```python
from build123d import *

# Parameters (mm, degrees)
BOSS_EXTRUDE1_DEPTH = 4.064


with BuildPart() as part:
    # Sketch1 → Boss-Extrude1 (new body)
    with BuildSketch(Plane(origin=(0, 0, 0), x_dir=(0, 0, -1), z_dir=(1, 0, 0))):
        Polygon((10.353307799, 10.287), (10.353307799, 0), (33.467307799, 0), (33.467307799, 2.413), (30.292307799, 2.413), (30.292307799, 3.937), (33.467307799, 3.937), (33.467307799, 7.493), (30.292307799, 7.493), (30.292307799, 10.287), align=None)
        Polygon((-12.760692201, 2.413), (-12.760692201, 0), (10.353307799, 0), (10.353307799, 10.287), (-9.585692201, 10.287), (-9.585692201, 7.493), (-12.760692201, 7.493), (-12.760692201, 3.937), (-9.585692201, 3.937), (-9.585692201, 2.413), align=None)
    extrude(amount=BOSS_EXTRUDE1_DEPTH)


solid = part.part
```
The listing builds one solid part. Answer for the finished solid, in the listing's coordinates (mm). A direction names the side the tool comes from. Coordinates: 2 decimals unless noted, no trailing zeros. Loops run counter-clockwise (first coordinate to the right, second up) from the corner with the lowest first, then second, coordinate; pieces in that order, holes last. Notation, with made-up numbers: (53, 55.25) - (65, 55.25) arc R18 ccw to (65, 78.25) - close; hole circle Ø2 at (-22.75, 18.5). An arc over 180 degrees is marked (long way). Use a Markdown table: item, result. Add a question column.
1) Find the intervals of material crossed by line 1 (Z direction, x = 3.35, y = 8), in increasing order.
2) The part is cut by section A-A, the plane x = 1.5. Give the vertices of the cut face in (y, z), and give its area (3 significant figures).
3) Given pin 1 (4 mm diameter, centred on y = 3.5, z = 1.5, fed in from -X); pin 2 (0.8 mm diameter, centred on x = 2.5, y = 3.5, fed in from -Z); pin 3 (0.5 mm diameter, centred on x = 2, y = 3, fed in from +Z); pin 4 (1 mm diameter, centred on x = 3, z = 11, fed in from +Y), each flat-ended and moving along its own axis, determine where each tip first touches the part or whether it passes through.
4) The mould has two halves that part along Y. Classify faces 1 (the flat face through (2, 9, 9.586)), 2 (the flat face through (2, 10.287, -11)), 3 (the flat face through (2, 3, 9.586)): released by +Y, released by -Y, zero draft, split by the parting line, or undercut.
5) For faces 4 (the flat face through (2, 7.493, 11)), 5 (the flat face through (2, 1, 12.761)), 6 (the flat face through (2, 2.413, 11)), 7 (the flat face through (2, 7.493, -32)), 8 (the flat face through (2, 3.937, -32)), determine the directions among +Z, -Z, +X, -X, +Y, -Y from which every point of the face is accessible in a straight line to the end or side of a thin tool.
Here are the results:
| question | item | result |
|---|---|---|
| 1 | line 1 | z = -30.29 to 9.59 |
| 2 | outline | (0, -33.47) - (2.41, -33.47) - (2.41, -30.29) - (3.94, -30.29) - (3.94, -33.47) - (7.49, -33.47) - (7.49, -30.29) - (10.29, -30.29) - (10.29, 9.59) - (7.49, 9.59) - (7.49, 12.76) - (3.94, 12.76) - (3.94, 9.59) - (2.41, 9.59) - (2.41, 12.76) - (0, 12.76) - close |
| 2 | area | 448 mm^2 |
| 3 | pin 1 | stops at x = 0 |
| 3 | pin 2 | stops at z = -30.29 |
| 3 | pin 3 | stops at z = 9.59 |
| 3 | pin 4 | stops at y = 7.49 |
| 4 | face 1 | zero draft |
| 4 | face 2 | released by +Y |
| 4 | face 3 | undercut |
| 5 | face 4 | +Z, +X, -X, +Y |
| 5 | face 5 | +Z, +X, -X, +Y, -Y |
| 5 | face 6 | +Z, +X, -X |
| 5 | face 7 | -Z, +X, -X, +Y |
| 5 | face 8 | -Z, +X, -X |
